from build123d import *

# Parameters (mm, degrees)
F0_W     = 50
F0_H     = 50
F1_DEPTH = 50
F2_R     = 11.6571142063
F3_DEPTH = 25
F4_R     = 10.382921487
F5_DEPTH = 25
F6_W     = 45.1483903453
F6_H     = 42.6243015099
F6_R     = 10.382921487
F7_DEPTH = 25
F8_R     = 11.4191364722
F9_DEPTH = 162


with BuildPart() as f1:
    # F0 (on Top) → F1 (new body)
    with BuildSketch(Plane.XY):
        with Locations((25, 25)):
            Rectangle(F0_W, F0_H)
    extrude(amount=F1_DEPTH)

    # F2 (on face) → F3 (join)
    with BuildSketch(Plane.XY.offset(50)):
        with Locations((12.9157425836, 30.8926273137)):
            Circle(F2_R)
    extrude(amount=F3_DEPTH)

    # F4 (on face) → F5 (join)
    with BuildSketch(Plane.XY.offset(50)):
        with Locations((32.7795855701, 14.4389113411)):
            Circle(F4_R)
    extrude(amount=F5_DEPTH)

    # F6 (on face) → F7 (join)
    with BuildSketch(Plane.XY.offset(75)):
        with Locations((20.978460554, 23.2780914521)):
            Rectangle(F6_W, F6_H)
        with Locations((32.7795855701, 14.4389113411)):
            Circle(F6_R, mode=Mode.SUBTRACT)
        with Locations((32.7795855701, 14.4389113411)):
            Circle(F6_R)
    extrude(amount=F7_DEPTH)

    # F8 (on face) → F9 (cut)
    with BuildSketch(Plane.XZ):
        with Locations((24.4850087911, 27.6993848383)):
            Circle(F8_R)
    extrude(amount=-F9_DEPTH, mode=Mode.SUBTRACT)


solid = f1.part
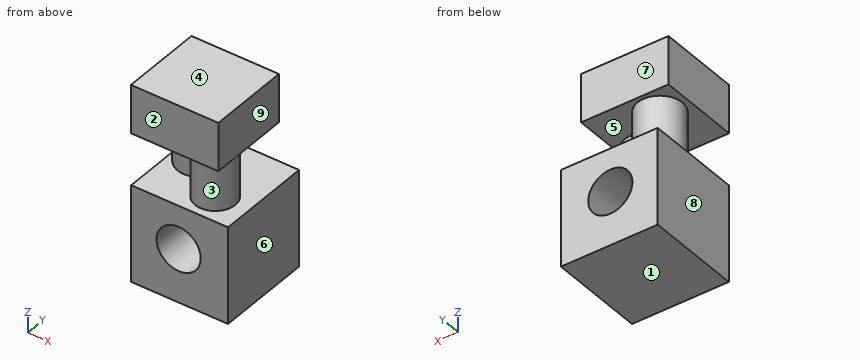
Check sheet for the modelled part. Datum: model origin and axes. Units: mm. Face numbers are marked on the shaded views. A direction names the side the tool comes from. Round coordinates to 2 decimals unless told otherwise and drop trailing zeros. Loops run counter-clockwise (first coordinate to the right, second up) from the corner with the lowest first, then second, coordinate; pieces in that order, holes last.
1. Sectioned sample at B-B on z = 32. Record the boundary of the cut face in (x, y).
2. Set-up check for the marked faces 5, 6, 7, 8 and 9: record each of +Z, -Z, +X, -X, +Y, -Y from which the full face is reachable in a straight line by a thin tool's end or side.
3. Sectioned sample at A-A on x = 28.5. Record the boundary of the cut face in (y, z).
4. Sectioned sample at D-D on y = 22.5. Record the boundary of the cut face in (x, z) (1 decimal), and give its area (3 significant figures).
5. Sectioned sample at C-C on y = 11.5. Record the boundary of the cut face in (x, z) (3 decimals).
6. Scan lines: probe 1 along Z at (x, y) = (31, 33); probe 2 along X at (y, z) = (27.5, 48); probe 3 along X at (y, z) = (41, 95.5). Record each from-to range of solid material in increasing order.
7. Gauge pin test, flat ends, axial feed: pin 1 Ø3 at (x, z) = (37, 69) entering from -Y; pin 2 Ø8 at (x, z) = (42.5, 75.5) entering from +Y; pin 3 Ø15 at (y, z) = (13, 13) entering from -X. Record the tip position at first contact, or that the pin passes through.
8. Mould release check, pull along Z, two halves, no side actions. Record for the marked faces 1, 2, 3 and 4: released by +Z, released by -Z, zero draft, split by the parting line, or undercut.
Recorded:
1. outline: (0, 0) - (13.91, 0) - (13.91, 50) - (0, 50) - close; (35.06, 0) - (50, 0) - (50, 50) - (35.06, 50) - close
2. face 5: none
2. face 6: +Z, -Z, +X, +Y, -Y
2. face 7: +Z, +X, -X, +Y
2. face 8: -Z, -X, +Y, -Y
2. face 9: +Z, +X, +Y, -Y
3. outline: (0, 0) - (50, 0) - (50, 17.01) - (0, 17.01) - close; (0, 38.39) - (50, 38.39) - (50, 50) - (23.9, 50) - (23.9, 75) - (44.59, 75) - (44.59, 100) - (1.97, 100) - (1.97, 75) - (4.98, 75) - (4.98, 50) - (0, 50) - close
4. outline: (-1.6, 75) - (4.8, 75) - (4.8, 50) - (0, 50) - (0, 0) - (50, 0) - (50, 50) - (39.3, 50) - (39.3, 75) - (43.6, 75) - (43.6, 100) - (-1.6, 100) - close; hole circle Ø22.8 at (24.5, 27.7); hole (21, 50) - (26.2, 50) - (26.2, 75) - (21, 75) - close
4. area: 3,950 mm2
5. outline: (-1.596, 75) - (22.821, 75) - (22.821, 50) - (0, 50) - (0, 0) - (50, 0) - (50, 50) - (42.738, 50) - (42.738, 75) - (43.553, 75) - (43.553, 100) - (-1.596, 100) - close; hole circle Ø22.838 at (24.485, 27.699)
6. probe 1: z = 0 to 18.32, 37.08 to 50, 75 to 100
6. probe 2: x = 0 to 50
6. probe 3: x = -1.6 to 43.55
7. pin 1: stops at y = 4.42
7. pin 2: stops at y = 44.59
7. pin 3: stops at x = 0
8. face 1: released by -Z
8. face 2: zero draft
8. face 3: undercut
8. face 4: released by +Z
